```python
from build123d import *

# Parameters (mm, degrees)
SKETCH1_R                                = 5
BOSS_EXTRUDE2_DEPTH                      = 82.55
CUT_EXTRUDE1_DEPTH                       = 2.54
TAP_DRILL_FOR_10_32_TAP1_D               = 4.0386
TAP_DRILL_FOR_10_32_TAP1_DEPTH           = 11.486682152
TAP_DRILL_FOR_10_32_TAP1_TIP             = 1.213317848
TAP_DRILL_FOR_10_32_TAP1_ON_FACE_2_D     = 4.0386
TAP_DRILL_FOR_10_32_TAP1_ON_FACE_2_DEPTH = 11.486682152
TAP_DRILL_FOR_10_32_TAP1_ON_FACE_2_TIP   = 1.213317848


with BuildPart() as part:
    # Sketch1 → Boss-Extrude2 (new body)
    with BuildSketch(Plane(origin=(0, 0, 0), x_dir=(1, 0, 0), z_dir=(0, 1, 0))):
        with Locations(Location((0, 0, 0), (0, 0, 270))):
            Circle(SKETCH1_R)
    extrude(amount=-BOSS_EXTRUDE2_DEPTH)

    # Sketch2 → Cut-Extrude1 (cut)
    with BuildSketch(Plane(origin=(0, 0, -5), x_dir=(-1, 0, 0), z_dir=(0, 0, -1))):
        with BuildLine():
            Line((-2, -109.22), (-2, -114.22))
            ThreePointArc((-2, -114.22), (0, -116.22), (2, -114.22))
            Line((2, -114.22), (2, -109.22))
            ThreePointArc((2, -109.22), (0, -107.22), (-2, -109.22))
        make_face()
        with BuildLine():
            Line((-1.5, -63.5), (-1.5, -68.5))
            ThreePointArc((-1.5, -68.5), (0, -70), (1.5, -68.5))
            Line((1.5, -68.5), (1.5, -63.5))
            ThreePointArc((1.5, -63.5), (0, -62), (-1.5, -63.5))
        make_face()
        with BuildLine():
            Line((-1.5, -10.39), (-1.5, -15.39))
            ThreePointArc((-1.5, -15.39), (0, -16.89), (1.5, -15.39))
            Line((1.5, -15.39), (1.5, -10.39))
            ThreePointArc((1.5, -10.39), (0, -8.89), (-1.5, -10.39))
        make_face()
    extrude(amount=-CUT_EXTRUDE1_DEPTH, mode=Mode.SUBTRACT)

    # Tap Drill for #10-32 Tap1
    with Locations(Plane.ZX):
        with Locations((0, 0)):
            Hole(TAP_DRILL_FOR_10_32_TAP1_D / 2, depth=TAP_DRILL_FOR_10_32_TAP1_DEPTH)
            with Locations((0, 0, -(TAP_DRILL_FOR_10_32_TAP1_DEPTH + TAP_DRILL_FOR_10_32_TAP1_TIP / 2))):  # 118° drill point
                Cone(0, TAP_DRILL_FOR_10_32_TAP1_D / 2, TAP_DRILL_FOR_10_32_TAP1_TIP, mode=Mode.SUBTRACT)

    # Tap Drill for #10-32 Tap1 on face 2
    with Locations(Plane(origin=(0, -82.55, 0), x_dir=(0, 0, -1), z_dir=(0, -1, 0))):
        with Locations((0, 0)):
            Hole(TAP_DRILL_FOR_10_32_TAP1_ON_FACE_2_D / 2, depth=TAP_DRILL_FOR_10_32_TAP1_ON_FACE_2_DEPTH)
            with Locations((0, 0, -(TAP_DRILL_FOR_10_32_TAP1_ON_FACE_2_DEPTH + TAP_DRILL_FOR_10_32_TAP1_ON_FACE_2_TIP / 2))):  # 118° drill point
                Cone(0, TAP_DRILL_FOR_10_32_TAP1_ON_FACE_2_D / 2, TAP_DRILL_FOR_10_32_TAP1_ON_FACE_2_TIP, mode=Mode.SUBTRACT)


solid = part.part
```
Input: part model. Units: mm. Frame: model coordinates. A direction names the side the tool comes from. Round coordinates to 2 decimals unless told otherwise and drop trailing zeros. Loops run counter-clockwise (first coordinate to the right, second up) from the corner with the lowest first, then second, coordinate; pieces in that order, holes last. Notation, with made-up numbers: M 51,2.25 L 87,2.25 A8 cw 87,13.25 Z; hole C 30.5,-35 d7. An arc over 180 degrees is marked long. Answer in a Markdown table with one row per item. Add a question column.
1. Ray query, probe 1 along Z at (x, y) = (0, -79); probe 2 along Y at (x, z) = (-1, -4). Return the intervals inside material, ascending.
2. Section B-B (x = 4). Output: boundary loops of the cut face in (y, z).
3. Contact query for flat-ended pins moving along their axis: pin 1 (2.5 mm diameter, centred on y = -67, z = -4, fed in from -X); pin 2 (1.2 mm diameter, centred on y = -65.5, z = -4, fed in from +X); pin 3 (1.5 mm diameter, centred on x = -0.5, y = -67, fed in from -Z). Output: stop coordinate, or through.
4. Section C-C (y = -14.5). Output: boundary loops of the cut face in (x, z), and give its area (3 significant figures).
5. Section A-A (y = -75). Output: boundary loops of the cut face in (x, z), and give its area (3 significant figures).
6. Set-up query: faces 4 (the face through (0.607, -76.726, 1.926)), 5 (the face through (0.03, -16.89, -3.75)), 6 (the face through (0.607, -5.824, -1.926)). Return all of +Z, -Z, +X, -X, +Y, -Y with unobstructed straight access to the full face (end or side cutting, diameter ignored); none if empty.
7. Mould query, pull axis Y, two halves, no side actions, for faces 1 (the face through (0.1, -82.55, 2.2)), 2 (the face through (0.1, 0, 2.2)), 3 (the face through (0, -13, -2.46)). Classes: released by +Y, released by -Y, zero draft, split by the parting line, or undercut.
Values follow:
| question | item | result |
|---|---|---|
| 1 | probe 1 | -5 to -2.02, 2.02 to 5 |
| 1 | probe 2 | -82.55 to -69.62, -62.38 to -16.51, -9.27 to 0 |
| 2 | outline | M -82.55,-3 L 0,-3 L 0,3 L -82.55,3 Z |
| 3 | pin 1 | x = -4.18 |
| 3 | pin 2 | x = 3.67 |
| 3 | pin 3 | z = -2.46 |
| 4 | outline | M -1.5,-4.77 L -1.5,-2.46 L 1.5,-2.46 L 1.5,-4.77 A5 ccw long Z |
| 4 | area | 71.1 mm^2 |
| 5 | outline | C 0,0 d10; hole C 0,0 d4.04 |
| 5 | area | 65.7 mm^2 |
| 6 | face 4 | -Y |
| 6 | face 5 | -Z |
| 6 | face 6 | +Y |
| 7 | face 1 | released by -Y |
| 7 | face 2 | released by +Y |
| 7 | face 3 | undercut |
